Build history of the part. All positions in model axes, mm. A direction names the side the tool comes from. Give positions to 0.01 mm unless a question says otherwise; leave off trailing zeros. Loops run counter-clockwise (first coordinate to the right, second up) from the corner with the lowest first, then second, coordinate; pieces in that order, holes last. Notation, with made-up numbers: (64, 25) -> (98, 25) arc R26 ccw to (98, 61) -> close; hole circle Ø10 at (9, -33.75). An arc over 180 degrees is marked (long way). One line per question, with ' | ' between items. Start each with the question number.
(1) Slice it at A-A, the plane z = 35.5. Write the cut outline in (x, y).
(2) Slice it at B-B, the plane x = -27. Write the cut outline in (y, z).
(3) Drill centre lines: L1, parallel to Y at x = -8.5, z = 42; L2, parallel to X at y = -36.5, z = 43; L3, parallel to Z at x = -14, y = -19. Where is each one in solid material? Low to high. Write a range as from..to.
(4) 3-axis set-ups, long thin cutter, end or side, ignore diameter. For faces 1 (the face through (0, -13, 45)), 2 (the face through (35, -35, 25)): which of +Z, -Z, +X, -X, +Y, -Y reach the whole face in a straight line?
(5) Slice it at C-C, the plane y = -38.5. Write the cut outline in (x, z), then the cut area to 3 significant figures.
(6) Flat gauge pin, fed straight in: pin 1 Ø8 at (x, y) = (19.5, -2.5) entering from +Z. Where does the tip first touch, or does it go through?
```python
from build123d import *

# Parameters (mm, degrees)
SKETCH1_W           = 80
SKETCH1_H           = 120
BOSS_EXTRUDE1_DEPTH = 5
SKETCH2_W           = 80
SKETCH2_H           = 120
SKETCH2_W_2         = 70
SKETCH2_H_2         = 66
SKETCH2_H_3         = 40
BOSS_EXTRUDE2_DEPTH = 40
FILLET1_R           = 5


with BuildPart() as part:
    # Sketch1 → Boss-Extrude1 (new body)
    with BuildSketch(Plane.XY):
        Rectangle(SKETCH1_W, SKETCH1_H)
    extrude(amount=BOSS_EXTRUDE1_DEPTH)

    # Sketch2 → Boss-Extrude2 (add)
    with BuildSketch(Plane.XY.offset(5)):
        Rectangle(SKETCH2_W, SKETCH2_H)
        with Locations((0, 22)):
            Rectangle(SKETCH2_W_2, SKETCH2_H_2, mode=Mode.SUBTRACT)
        with Locations((0, -35)):
            Rectangle(SKETCH2_W_2, SKETCH2_H_3, mode=Mode.SUBTRACT)
    extrude(amount=BOSS_EXTRUDE2_DEPTH)

    # Fillet1
    fillet1_edges = [part.edges().sort_by_distance(p)[0] for p in [
        (40, -60, 22.5),
        (-40, -60, 22.5),
        (-40, 60, 22.5),
        (40, 60, 22.5),
    ]]
    fillet(fillet1_edges, radius=FILLET1_R)


solid = part.part
```
Final values:
1) outline: (-40, -55) arc R5 ccw to (-35, -60) -> (35, -60) arc R5 ccw to (40, -55) -> (40, 55) arc R5 ccw to (35, 60) -> (-35, 60) arc R5 ccw to (-40, 55) -> close; hole (-35, -55) -> (35, -55) -> (35, -15) -> (-35, -15) -> close; hole (-35, -11) -> (35, -11) -> (35, 55) -> (-35, 55) -> close
2) outline: (-60, 0) -> (60, 0) -> (60, 45) -> (55, 45) -> (55, 5) -> (-11, 5) -> (-11, 45) -> (-15, 45) -> (-15, 5) -> (-55, 5) -> (-55, 45) -> (-60, 45) -> close
3) L1: -60..-55, -15..-11, 55..60 | L2: -40..-35, 35..40 | L3: 0..5
4) face 1: +Z, +X, -X, +Y, -Y | face 2: +Z
5) outline: (-40, 0) -> (40, 0) -> (40, 45) -> (35, 45) -> (35, 5) -> (-35, 5) -> (-35, 45) -> (-40, 45) -> close | area: 800 mm2
6) pin 1: z = 5
